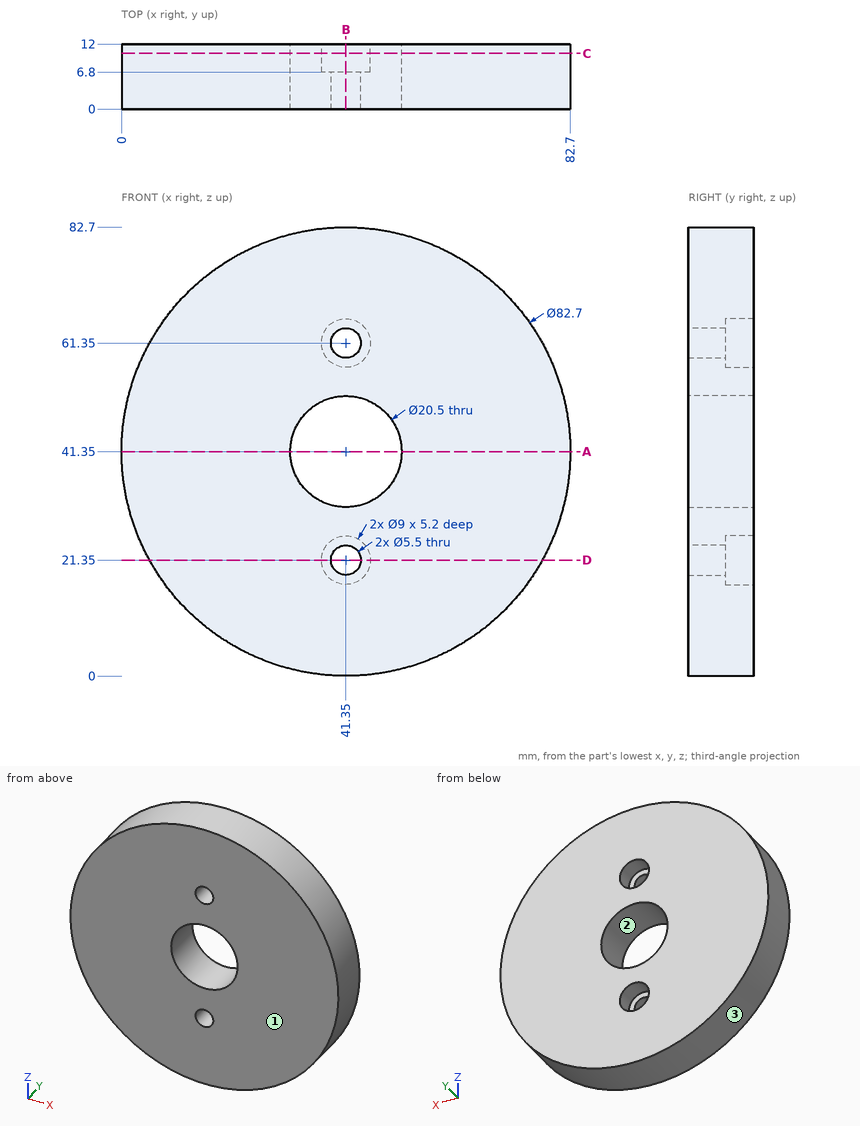
Answer from the drawing. Dimensions are ordinates in mm from the lowest x, y and z of the part. Coordinates: 2 decimals unless noted, no trailing zeros. Loops run counter-clockwise (first coordinate to the right, second up) from the corner with the lowest first, then second, coordinate; pieces in that order, holes last. Notation, with made-up numbers: (-14, 48.5) -> (-6, 48.5) arc R22 ccw to (-6, 65.5) -> close; hole circle Ø7 at (-19.75, -12). An arc over 180 degrees is marked (long way). Return JSON: item names as keys, results as strings.
Item 1: Find the intervals of material crossed by probe 1 along X at (y, z) = (1.5, 61.35); probe 2 along X at (y, z) = (3.5, 62.5); probe 3 along X at (y, z) = (7.5, 28), in increasing order.
Answers:
{"probe 1": "x = 5.16 to 38.6, 44.1 to 77.54", "probe 2": "x = 5.82 to 38.85, 43.85 to 76.88", "probe 3": "x = 2.21 to 80.49"}
Item 2: Flat-ended cylindrical pins translate along their axes: P1, Ø1, axis at y = 1, z = 15, coming from the +X side; P2, Ø4, axis at x = 50, y = 7, coming from the -Z side; P3, Ø2.5, axis at x = 42, z = 62.5, coming from the +Y side; P4, Ø4, axis at y = 4, z = 72, coming from the +X side. Find the tip coordinate at first contact, or state that the pin passes through.
Answers:
{"P1": "stops at x = 73.62", "P2": "stops at z = 0.54", "P3": "passes through", "P4": "stops at x = 71.17"}
Item 3: Find section A-A (z = 41.35). Determine the outline of the cut face in (x, y).
Answers:
{"outline": "(0, 0) -> (31.1, 0) -> (31.1, 12) -> (0, 12) -> close; (51.6, 0) -> (82.7, 0) -> (82.7, 12) -> (51.6, 12) -> close"}
Item 4: Find section B-B (x = 41.35). Determine the outline of the cut face in (y, z), plus the area to 3 significant figures.
Answers:
{"outline": "(0, 0) -> (12, 0) -> (12, 16.85) -> (6.8, 16.85) -> (6.8, 18.6) -> (0, 18.6) -> close; (0, 24.1) -> (6.8, 24.1) -> (6.8, 25.85) -> (12, 25.85) -> (12, 31.1) -> (0, 31.1) -> close; (0, 51.6) -> (12, 51.6) -> (12, 56.85) -> (6.8, 56.85) -> (6.8, 58.6) -> (0, 58.6) -> close; (0, 64.1) -> (6.8, 64.1) -> (6.8, 65.85) -> (12, 65.85) -> (12, 82.7) -> (0, 82.7) -> close", "area": "578 mm2"}
Item 5: Find section C-C (y = 10.25). Determine the outline of the cut face in (x, z), plus the area to 3 significant figures.
Answers:
{"outline": "circle Ø82.7 at (41.35, 41.35); hole circle Ø20.5 at (41.35, 41.35); hole circle Ø9 at (41.35, 21.35); hole circle Ø9 at (41.35, 61.35)", "area": "4,910 mm2"}
Item 6: For a pull along X with two mould halves and no side action, classify the marked faces 1, 2 and 3 as +X half, -X half, draft (parallel to the pull), parting line (faces both ways), or undercut.
Answers:
{"face 1": "draft", "face 2": "undercut", "face 3": "parting line"}
Item 7: Find section D-D (z = 21.35). Determine the outline of the cut face in (x, y).
Answers:
{"outline": "(5.16, 0) -> (38.6, 0) -> (38.6, 6.8) -> (36.85, 6.8) -> (36.85, 12) -> (5.16, 12) -> close; (44.1, 0) -> (77.54, 0) -> (77.54, 12) -> (45.85, 12) -> (45.85, 6.8) -> (44.1, 6.8) -> close"}
